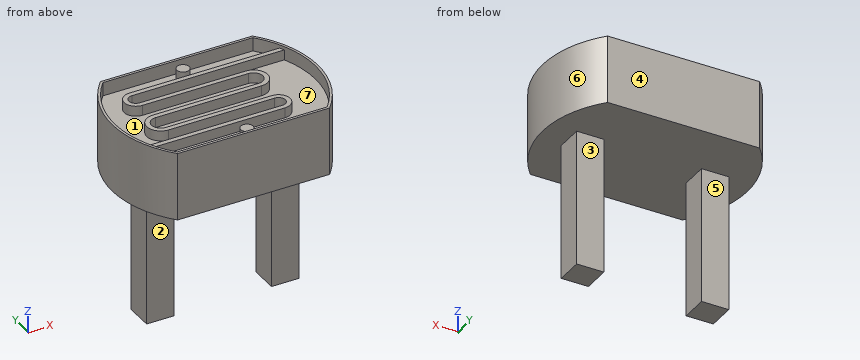
```python
from build123d import *

# Parameters (mm, degrees)
BOSS_EXTRUDE1_DEPTH = 8
SKETCH2_W           = 4
SKETCH2_H           = 4
BOSS_EXTRUDE2_DEPTH = 20
BOSS_EXTRUDE3_DEPTH = 2
SKETCH4_R           = 0.91109378
BOSS_EXTRUDE4_DEPTH = 1.5


with BuildPart() as part:
    # Sketch1 → Boss-Extrude1 (new body)
    with BuildSketch(Plane.XY):
        with BuildLine():
            Line((-11.180339887, 10), (11.180339887, 10))
            ThreePointArc((11.180339887, 10), (15, 0), (11.180339887, -10))
            Line((11.180339887, -10), (-11.180339887, -10))
            ThreePointArc((-11.180339887, -10), (-15, 0), (-11.180339887, 10))
        make_face()
    extrude(amount=BOSS_EXTRUDE1_DEPTH)

    # Sketch2 → Boss-Extrude2 (add)
    with BuildSketch(Plane(origin=(0, 0, 0), x_dir=(-1, 0, 0), z_dir=(0, 0, -1))):
        with Locations((-9.180339887, 0)):
            Rectangle(SKETCH2_W, SKETCH2_H)
        Polygon((7.180339887, 2), (7.180339887, -2), (11.180339887, -2), (11.180339887, 0), (11.180339887, 2), align=None)
    extrude(amount=BOSS_EXTRUDE2_DEPTH)

    # Sketch3 → Boss-Extrude3 (add)
    with BuildSketch(Plane.XY.offset(8)):
        with BuildLine():
            Line((-11.180339887, -10), (11.180339887, -10))
            ThreePointArc((11.180339887, -10), (15, 0), (11.180339887, 10))
            Line((11.180339887, 10), (-11.180339887, 10))
            ThreePointArc((-11.180339887, 10), (-15, 0), (-11.180339887, -10))
        make_face()
        with BuildLine():
            ThreePointArc((-11.021413403, 9.634230221), (-14.638645612, 0), (-11.021413403, -9.634230221))
            Line((-11.021413403, -9.634230221), (11.021413403, -9.634230221))
            ThreePointArc((11.021413403, -9.634230221), (14.638645612, 0), (11.021413403, 9.634230221))
            Line((11.021413403, 9.634230221), (-11.021413403, 9.634230221))
        make_face(mode=Mode.SUBTRACT)
    extrude(amount=BOSS_EXTRUDE3_DEPTH)

    # Sketch4 → Boss-Extrude4 (add)
    with BuildSketch(Plane.XY.offset(8)):
        with Locations((0, 8.266858506)):
            Circle(SKETCH4_R)
        with Locations(Location((0, -8.266858506, 0), (0, 0, 180))):
            Circle(SKETCH4_R)
        with BuildLine():
            Line((13.1358141, 6.460675915), (-8.940009027, 6.460675915))
            ThreePointArc((-8.940009027, 6.460675915), (-10.640009027, 4.760675915), (-8.940009027, 3.060675915))
            Line((-8.940009027, 3.060675915), (6.638090535, 3.060675915))
            ThreePointArc((6.638090535, 3.060675915), (7.993428493, 1.705337957), (6.638090535, 0.35))
            Line((6.638090535, 0.35), (-8.940009027, 0.35))
            ThreePointArc((-8.940009027, 0.35), (-10.995346985, -1.705337957), (-8.940009027, -3.760675915))
            Line((-8.940009027, -3.760675915), (6.638090535, -3.760675915))
            ThreePointArc((6.638090535, -3.760675915), (7.638090535, -4.760675915), (6.638090535, -5.760675915))
            Line((6.638090535, -5.760675915), (-8.940009027, -5.760675915))
            Line((-8.940009027, -5.760675915), (-13.457509367, -5.760675915))
            ThreePointArc((-13.457509367, -5.760675915), (-13.301267355, -6.112792496), (-13.1358141, -6.460675915))
            Line((-13.1358141, -6.460675915), (-8.940009027, -6.460675915))
            Line((-8.940009027, -6.460675915), (6.638090535, -6.460675915))
            ThreePointArc((6.638090535, -6.460675915), (8.338090535, -4.760675915), (6.638090535, -3.060675915))
            Line((6.638090535, -3.060675915), (-8.940009027, -3.060675915))
            ThreePointArc((-8.940009027, -3.060675915), (-10.295346985, -1.705337957), (-8.940009027, -0.35))
            Line((-8.940009027, -0.35), (6.638090535, -0.35))
            ThreePointArc((6.638090535, -0.35), (8.693428493, 1.705337957), (6.638090535, 3.760675915))
            Line((6.638090535, 3.760675915), (-8.940009027, 3.760675915))
            ThreePointArc((-8.940009027, 3.760675915), (-9.940009027, 4.760675915), (-8.940009027, 5.760675915))
            Line((-8.940009027, 5.760675915), (13.457509367, 5.760675915))
            ThreePointArc((13.457509367, 5.760675915), (13.301267355, 6.112792496), (13.1358141, 6.460675915))
        make_face()
    extrude(amount=BOSS_EXTRUDE4_DEPTH)


solid = part.part
```
Input: part model. Units: mm. Frame: model coordinates. Face numbers are marked on the shaded views. A direction names the side the tool comes from. Give positions to 0.01 mm unless a question says otherwise; leave off trailing zeros. Order: outer loops, then holes, each group sorted by start corner. A loop starts at its lowest first (then second) coordinate and runs counter-clockwise, first axis right, second up.
1. Cut plane B-B (x = -3.5). Return loops of the section in (y, z).
Computed:
outline: (-10, 0) - (10, 0) - (10, 10) - (9.63, 10) - (9.63, 8) - (6.46, 8) - (6.46, 9.5) - (5.76, 9.5) - (5.76, 8) - (3.76, 8) - (3.76, 9.5) - (3.06, 9.5) - (3.06, 8) - (0.35, 8) - (0.35, 9.5) - (-0.35, 9.5) - (-0.35, 8) - (-3.06, 8) - (-3.06, 9.5) - (-3.76, 9.5) - (-3.76, 8) - (-5.76, 8) - (-5.76, 9.5) - (-6.46, 9.5) - (-6.46, 8) - (-9.63, 8) - (-9.63, 10) - (-10, 10) - close
2. Draft query along X for the marked faces 5, 6 and 7. Return one class per face: released by +X, released by -X, zero draft, split by the parting line, or undercut.
Computed:
face 5: zero draft
face 6: released by +X
face 7: undercut
3. Cut plane C-C (x = -11.75). Return loops of the section in (y, z).
Computed:
outline: (-9.32, 0) - (9.32, 0) - (9.32, 10) - (8.73, 10) - (8.73, 8) - (-5.76, 8) - (-5.76, 9.5) - (-6.46, 9.5) - (-6.46, 8) - (-8.73, 8) - (-8.73, 10) - (-9.32, 10) - close
4. Set-up query: the marked faces 1, 2, 3 and 4. Return all of +Z, -Z, +X, -X, +Y, -Y with unobstructed straight access to the full face (end or side cutting, diameter ignored); none if empty.
Computed:
face 1: +Z
face 2: -Z, +X, -X, -Y
face 3: -Z, +X, -X, +Y
face 4: +Z, -Z, +X, -X, +Y
5. Cut plane A-A (z = -14.25). Return loops of the section in (x, y).
Computed:
outline: (-11.18, -2) - (-7.18, -2) - (-7.18, 2) - (-11.18, 2) - close; (7.18, -2) - (11.18, -2) - (11.18, 2) - (7.18, 2) - close
6. Pin query (flat end, axial travel): pin 1 Ø2 at (x, y) = (0.5, 8) entering from +Z; pin 2 Ø10 at (y, z) = (-2.5, -14.5) entering from -X; pin 3 Ø10 at (y, z) = (5, -3) entering from -X. Return the tip coordinate at first contact, or that it passes through.
Computed:
pin 1: stops at z = 9.5
pin 2: stops at x = -11.18
pin 3: stops at x = -14.97
7. Line query: probe 1 along X at (y, z) = (-1.75, -1.5); probe 2 along Y at (x, z) = (-11.5, 8.75); probe 3 along Y at (x, z) = (8, -12.75). Output: solid intervals per line, ascending.
Computed:
probe 1: x = -11.18 to -7.18, 7.18 to 11.18
probe 2: y = -9.63 to -9.06, -6.46 to -5.76, 9.06 to 9.63
probe 3: y = -2 to 2
